Study the drawing (mm; zero at the part's minimum x, y, z) and answer. Give positions to 0.01 mm unless a question says otherwise; leave off trailing zeros. Order: outer loops, then holes, each group sorted by start corner. A loop starts at its lowest first (then second) coordinate and runs counter-clockwise, first axis right, second up.
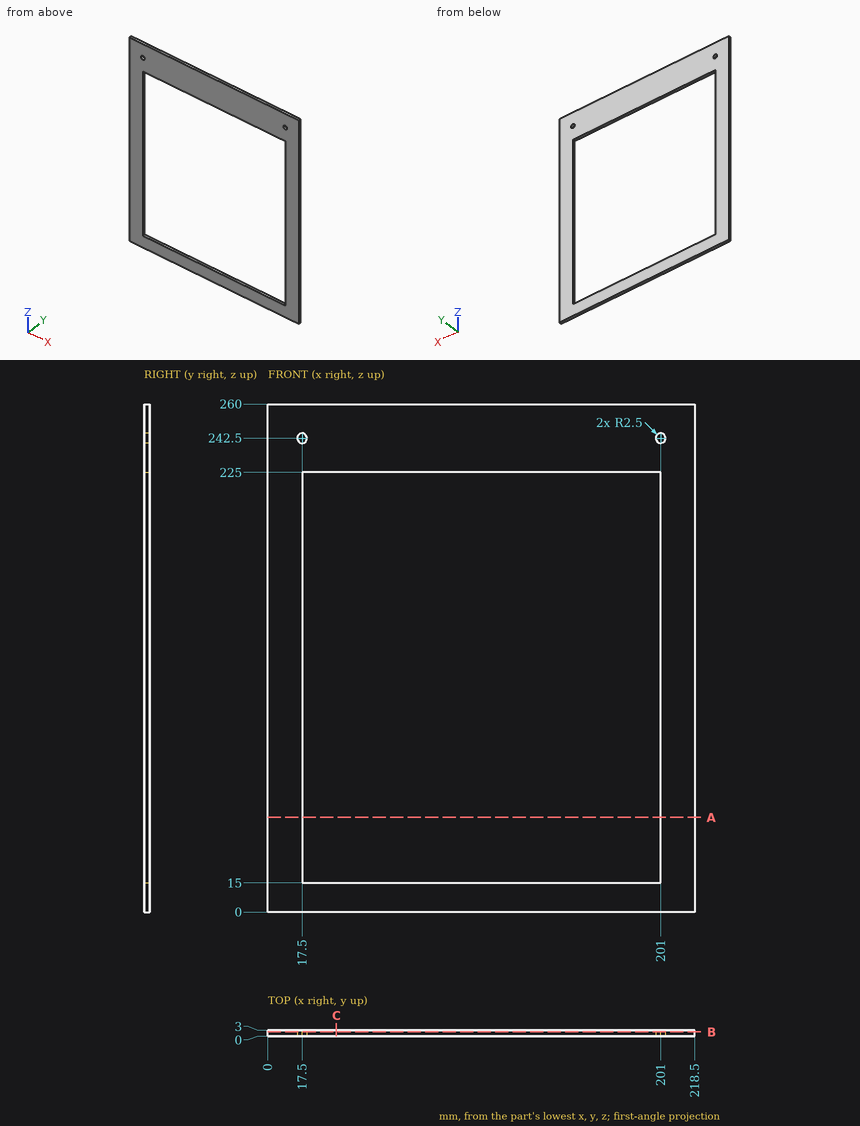
1) Find section C-C (x = 35). Write down the section's boundary in (y, z), then the cut area to 3 significant figures.
Geometry says:
outline: (0, 0) - (3, 0) - (3, 15) - (0, 15) - close; (0, 225) - (3, 225) - (3, 260) - (0, 260) - close
area: 150 mm2
2) Straight lines are drawn through the part: probe 1 along Z at (x, y) = (73.5, 0.35); probe 2 along X at (y, z) = (0.5, 191); probe 3 along Z at (x, y) = (16.5, 1.5). For each, find the intervals that lie inside material, in ascending order.
Geometry says:
probe 1: z = 0 to 15, 225 to 260
probe 2: x = 0 to 17.5, 201 to 218.5
probe 3: z = 0 to 240.21, 244.79 to 260
3) Find section A-A (z = 48.5). Write down the section's boundary in (x, y).
Geometry says:
outline: (0, 0) - (17.5, 0) - (17.5, 3) - (0, 3) - close; (201, 0) - (218.5, 0) - (218.5, 3) - (201, 3) - close
4) Find section B-B (y = 2.1). Write down the section's boundary in (x, z), then the cut area to 3 significant figures.
Geometry says:
outline: (0, 0) - (218.5, 0) - (218.5, 260) - (0, 260) - close; hole circle Ø5 at (17.5, 242.5); hole (17.5, 15) - (201, 15) - (201, 225) - (17.5, 225) - close; hole circle Ø5 at (201, 242.5)
area: 18,200 mm2
